The model under review builds one solid part; all positions refer to its coordinate system, in mm. A direction names the side the tool comes from. Coordinates: 2 decimals unless noted, no trailing zeros. Order: outer loops, then holes, each group sorted by start corner. A loop starts at its lowest first (then second) coordinate and runs counter-clockwise, first axis right, second up. Notation, with made-up numbers: M 18.5,29.25 L 42.5,29.25 A12 cw 42.5,41.25 Z; hole C 76,33 d9. An arc over 180 degrees is marked long. Write each question's results on one line, items separated by ' | '.
from build123d import *

# Parameters (mm, degrees)
SKETCH1_W           = 149.5
SKETCH1_H           = 70
BOSS_EXTRUDE1_DEPTH = 8
FILLET1_R           = 4
SKETCH6_W           = 147
SKETCH6_H           = 67.5
BOSS_EXTRUDE3_DEPTH = 5
FILLET2_R           = 4
SKETCH7_W           = 6.205469591
SKETCH7_H           = 30
BOSS_EXTRUDE4_DEPTH = 7
SKETCH8_R           = 1
CUT_EXTRUDE3_DEPTH  = 154.632882223
FILLET5_R           = 4
SKETCH9_W           = 90
SKETCH9_H           = 56
CUT_EXTRUDE4_DEPTH  = 7
SKETCH10_W          = 79
SKETCH10_H          = 56
CUT_EXTRUDE5_DEPTH  = 4
SKETCH11_W          = 66
SKETCH11_H          = 50
CUT_EXTRUDE6_DEPTH  = 85.478177656
SKETCH13_W          = 6
SKETCH13_H          = 50
BOSS_EXTRUDE5_DEPTH = 4
SKETCH14_R          = 1.692809378
CUT_EXTRUDE7_DEPTH  = 85.270768953
SKETCH15_W          = 6
SKETCH15_H          = 30
CUT_EXTRUDE8_DEPTH  = 2
CHAMFER2_SIZE       = 2
SKETCH16_R          = 3.75
CUT_EXTRUDE9_DEPTH  = 84.555744865
SKETCH17_W          = 12.5
SKETCH17_H          = 12.5
CUT_EXTRUDE10_DEPTH = 8
SKETCH20_W          = 24
SKETCH20_H          = 4
CUT_EXTRUDE12_DEPTH = 8
FILLET6_R           = 4
CHAMFER3_SIZE       = 2
SKETCH23_W          = 5.5
SKETCH23_H          = 43
CUT_EXTRUDE15_DEPTH = 4
FILLET7_R           = 1.5
CHAMFER6_SIZE       = 2
SKETCH26_W          = 27.5
SKETCH26_H          = 20
CUT_EXTRUDE16_DEPTH = 10
SKETCH27_W          = 27.410939183
SKETCH27_H          = 28.83766823
CUT_EXTRUDE17_DEPTH = 5
CHAMFER7_SIZE       = 3


with BuildPart() as part:
    # Sketch1 → Boss-Extrude1 (new body)
    with BuildSketch(Plane(origin=(0, 0, 0), x_dir=(1, 0, 0), z_dir=(0, 1, 0))):
        Rectangle(SKETCH1_W, SKETCH1_H)
    extrude(amount=BOSS_EXTRUDE1_DEPTH)

    # Fillet1
    fillet1_edges = [part.edges().sort_by_distance(p)[0] for p in [
        (74.75, 4, 35),
        (-74.75, 4, 35),
        (-74.75, 4, -35),
        (74.75, 4, -35),
    ]]
    fillet(fillet1_edges, radius=FILLET1_R)

    # Sketch6 → Boss-Extrude3 (add)
    with BuildSketch(Plane(origin=(0, 8, 0), x_dir=(1, 0, 0), z_dir=(0, 1, 0))):
        Rectangle(SKETCH6_W, SKETCH6_H)
    extrude(amount=BOSS_EXTRUDE3_DEPTH)

    # Fillet2
    fillet2_edges = [part.edges().sort_by_distance(p)[0] for p in [
        (73.5, 10.5, 33.75),
        (73.5, 10.5, -33.75),
        (-73.5, 10.5, -33.75),
        (-73.5, 10.5, 33.75),
    ]]
    fillet(fillet2_edges, radius=FILLET2_R)

    # Sketch7 → Boss-Extrude4 (add)
    with BuildSketch(Plane(origin=(0, 13, 0), x_dir=(1, 0, 0), z_dir=(0, 1, 0))):
        with Locations((-70.397265205, 0)):
            Rectangle(SKETCH7_W, SKETCH7_H)
        with Locations((70.397265205, 0)):
            Rectangle(SKETCH7_W, SKETCH7_H)
    extrude(amount=BOSS_EXTRUDE4_DEPTH)

    # Sketch8 → Cut-Extrude3 (cut, through all)
    with BuildSketch(Plane.ZY.offset(73.5)):
        with Locations((-7, 16)):
            Circle(SKETCH8_R)
        with Locations((7, 16)):
            Circle(SKETCH8_R)
    extrude(amount=-CUT_EXTRUDE3_DEPTH, mode=Mode.SUBTRACT)

    # Fillet5
    fillet5_edges = [part.edges().sort_by_distance(p)[0] for p in [
        (-70.397265204, 20, 15),
        (-70.397265204, 20, -15),
        (70.397265204, 20, -15),
        (70.397265204, 20, 15),
    ]]
    fillet(fillet5_edges, radius=FILLET5_R)

    # Sketch9 → Cut-Extrude4 (cut)
    with BuildSketch(Plane(origin=(0, 13, 0), x_dir=(1, 0, 0), z_dir=(0, 1, 0))):
        with Locations((-22, 0)):
            Rectangle(SKETCH9_W, SKETCH9_H)
    extrude(amount=-CUT_EXTRUDE4_DEPTH, mode=Mode.SUBTRACT)

    # Sketch10 → Cut-Extrude5 (cut)
    with BuildSketch(Plane(origin=(0, 6, 0), x_dir=(1, 0, 0), z_dir=(0, 1, 0))):
        with Locations((-22, 0)):
            Rectangle(SKETCH10_W, SKETCH10_H)
    extrude(amount=-CUT_EXTRUDE5_DEPTH, mode=Mode.SUBTRACT)

    # Sketch11 → Cut-Extrude6 (cut, through all)
    with BuildSketch(Plane(origin=(0, 2, 0), x_dir=(1, 0, 0), z_dir=(0, 1, 0))):
        with Locations((-18.5, 0)):
            Rectangle(SKETCH11_W, SKETCH11_H)
    extrude(amount=-CUT_EXTRUDE6_DEPTH, mode=Mode.SUBTRACT)

    # Sketch13 → Boss-Extrude5 (add)
    with BuildSketch(Plane(origin=(0, 13, 0), x_dir=(1, 0, 0), z_dir=(0, 1, 0))):
        with Locations((26, 0)):
            Rectangle(SKETCH13_W, SKETCH13_H)
    extrude(amount=BOSS_EXTRUDE5_DEPTH)

    # Sketch14 → Cut-Extrude7 (cut, through all)
    with BuildSketch(Plane(origin=(0, 17, 0), x_dir=(1, 0, 0), z_dir=(0, 1, 0))):
        with Locations(Location((26, 20, 0), (0, 0, 270))):
            Circle(SKETCH14_R)
        with Locations(Location((26, -20, 0), (0, 0, 90))):
            Circle(SKETCH14_R)
    extrude(amount=-CUT_EXTRUDE7_DEPTH, mode=Mode.SUBTRACT)

    # Sketch15 → Cut-Extrude8 (cut)
    with BuildSketch(Plane(origin=(0, 17, 0), x_dir=(1, 0, 0), z_dir=(0, 1, 0))):
        with Locations((26, 0)):
            Rectangle(SKETCH15_W, SKETCH15_H)
    extrude(amount=-CUT_EXTRUDE8_DEPTH, mode=Mode.SUBTRACT)

    # Chamfer2
    chamfer2_edges = [part.edges().sort_by_distance(p)[0] for p in [
        (26, 0, -21.692809378),
        (26, 0, 21.692809378),
    ]]
    chamfer(chamfer2_edges, length=CHAMFER2_SIZE)

    # Sketch16 → Cut-Extrude9 (cut, through all)
    with BuildSketch(Plane(origin=(0, 13, 0), x_dir=(1, 0, 0), z_dir=(0, 1, 0))):
        with Locations(Location((49.294530409, 0, 0), (0, 0, 270))):
            Circle(SKETCH16_R)
    extrude(amount=-CUT_EXTRUDE9_DEPTH, mode=Mode.SUBTRACT)

    # Sketch17 → Cut-Extrude10 (cut)
    with BuildSketch(Plane(origin=(0, 13, 0), x_dir=(1, 0, 0), z_dir=(0, 1, 0))):
        with Locations((49.294530409, 0)):
            Rectangle(SKETCH17_W, SKETCH17_H)
    extrude(amount=-CUT_EXTRUDE10_DEPTH, mode=Mode.SUBTRACT)

    # Sketch20 → Cut-Extrude12 (cut)
    with BuildSketch(Plane(origin=(0, 13, 0), x_dir=(1, 0, 0), z_dir=(0, 1, 0))):
        with Locations((-22, 30)):
            Rectangle(SKETCH20_W, SKETCH20_H)
        with Locations((-22, -30)):
            Rectangle(SKETCH20_W, SKETCH20_H)
    extrude(amount=-CUT_EXTRUDE12_DEPTH, mode=Mode.SUBTRACT)

    # Fillet6
    fillet6_edges = [part.edges().sort_by_distance(p)[0] for p in [
        (-34, 9, 32),
        (-10, 9, 32),
        (-10, 9, -32),
        (-34, 9, -32),
    ]]
    fillet(fillet6_edges, radius=FILLET6_R - 0.0001)  # a hair under: the kernel refuses the full size

    # Chamfer3
    chamfer3_edges = [part.edges().sort_by_distance(p)[0] for p in [
        (26, 17, 15),
        (26, 17, -15),
        (26, 17, -25),
        (26, 17, 25),
    ]]
    chamfer(chamfer3_edges, length=CHAMFER3_SIZE - 0.0001)  # a hair under: the kernel refuses the full size

    # Sketch23 → Cut-Extrude15 (cut)
    with BuildSketch(Plane(origin=(0, 6, 0), x_dir=(1, 0, 0), z_dir=(0, 1, 0))):
        with Locations((-64.25, 0)):
            Rectangle(SKETCH23_W, SKETCH23_H)
        with Locations((20.25, 0)):
            Rectangle(SKETCH23_W, SKETCH23_H)
    extrude(amount=-CUT_EXTRUDE15_DEPTH, mode=Mode.SUBTRACT)

    # Fillet7
    fillet7_edges = [part.edges().sort_by_distance(p)[0] for p in [
        (14.5, 1, -25),
        (14.5, 1, 25),
        (-51.5, 1, 25),
        (-51.5, 1, -25),
    ]]
    fillet(fillet7_edges, radius=FILLET7_R)

    # Chamfer6
    chamfer6_edges = [part.edges().sort_by_distance(p)[0] for p in [
        (-61.5, 4, 21.5),
        (-61.5, 4, -21.5),
        (17.5, 4, 21.5),
        (17.5, 4, -21.5),
    ]]
    chamfer(chamfer6_edges, length=CHAMFER6_SIZE)

    # Sketch26 → Cut-Extrude16 (cut)
    with BuildSketch(Plane(origin=(0, 13, 0), x_dir=(1, 0, 0), z_dir=(0, 1, 0))):
        with Locations((49.25, -21.75)):
            Rectangle(SKETCH26_W, SKETCH26_H)
        with Locations((49.25, 21.75)):
            Rectangle(SKETCH26_W, SKETCH26_H)
    extrude(amount=-CUT_EXTRUDE16_DEPTH, mode=Mode.SUBTRACT)

    # Sketch27 → Cut-Extrude17 (cut)
    with BuildSketch(Plane(origin=(0, 13, 0), x_dir=(1, 0, 0), z_dir=(0, 1, 0))):
        with Locations((49.294530409, 0)):
            Rectangle(SKETCH27_W, SKETCH27_H)
    extrude(amount=-CUT_EXTRUDE17_DEPTH, mode=Mode.SUBTRACT)

    # Chamfer7
    chamfer7_edges = [part.edges().sort_by_distance(p)[0] for p in [
        (-74.75, 0, 0),
        (74.75, 0, 0),
        (0, 0, 35),
        (0, 0, -35),
        (73.578427125, 0, 33.828427125),
        (73.578427125, 0, -33.828427125),
        (-73.578427125, 0, 33.828427125),
        (-73.578427125, 0, -33.828427125),
    ]]
    chamfer(chamfer7_edges, length=CHAMFER7_SIZE)


solid = part.part
1) Take a section at A-A on z = 20. Count the separate pieces of the cut face and the enclosed holes in it, plus the area to 3 significant figures.
Solutions:
separate pieces: 3 | enclosed holes: 0 | area: 487 mm2
2) For pin 1 (4 mm diameter, centred on x = -35.5, z = 25.5, fed in from +Y); pin 2 (1.5 mm diameter, centred on x = -22, y = 9.5, fed in from +Z); pin 3 (5 mm diameter, centred on y = 9.5, z = -10, fed in from -X); pin 4 (2 mm diameter, centred on x = 25, z = -16.5, fed in from +Y), all flat-tipped, find the tip position at first contact; note any pin that passes through.
Solutions:
pin 1: y = 2 | pin 2: z = 33.75 | pin 3: x = -74.75 | pin 4: y = 17
3) Take a section at B-B on x = -47. State the section outline as (y, z) points, plus the area to 4 significant figures.
Solutions:
outline: M 0,-32 L 3,-35 L 8,-35 L 8,-33.75 L 13,-33.75 L 13,-28 L 2,-28 L 2,-25 L 0,-25 Z; M 0,25 L 2,25 L 2,28 L 13,28 L 13,33.75 L 8,33.75 L 8,35 L 3,35 L 0,32 Z | area: 172.5 mm2
4) Take a section at D-D on x = -28. State the section outline as (y, z) points, plus the area to 4 significant figures.
Solutions:
outline: M 0,-32 L 3,-35 L 8,-35 L 8,-33.75 L 13,-33.75 L 13,-32 L 5,-32 L 5,-28 L 2,-28 L 2,-25 L 0,-25 Z; M 0,25 L 2,25 L 2,28 L 5,28 L 5,32 L 13,32 L 13,33.75 L 8,33.75 L 8,35 L 3,35 L 0,32 Z | area: 108.5 mm2
5) The part is to be moulded in two halves that separate along X. For faces 1 (the flat face through (-1, 5, 35)), 2 (the cylindrical face through (-73.609, 5.535, -33.797)), 3 (the flat face through (-67, 8, 0)), say which applies: pulls with the +X half, pulls with the -X half, needs draft (parallel to the pull), parting line crosses it, or undercut.
Solutions:
face 1: needs draft | face 2: pulls with the -X half | face 3: undercut
6) Take a section at C-C on x = 32.5. State the section outline as (y, z) points, plus the area to 4 significant figures.
Solutions:
outline: M 0,-32 L 3,-35 L 8,-35 L 8,-33.75 L 13,-33.75 L 13,33.75 L 8,33.75 L 8,35 L 3,35 L 0,32 Z | area: 888.5 mm2
7) For faces 4 (the flat face through (73.5, 13, 0)), 5 (the flat face through (26, 15, 0)), 6 (the conical face through (72.55, 1.52, 32.76)), list the 3-axis set-ups (+Z, -Z, +X, -X, +Y, -Y) from which the entire face can be reached by the end or side of a thin tool; tool diameter is ignored.
Solutions:
face 4: +Z, -Z, +X, +Y | face 5: +Y | face 6: +Z, +X, -Y
8) To check wall thickness, follow line 1 along X through (y, z) = (14.75, 14); line 2 along X through (y, z) = (12, -0.5); line 3 along X through (y, z) = (9, -20). State the ranges of each line that lie inside material, in increasing order.
Solutions:
line 1: -73.5 to -67.29, 23 to 29, 67.29 to 73.5 | line 2: -73.5 to -67, 23 to 35.59, 63 to 73.5 | line 3: -73.5 to -67, 23 to 24.31, 27.69 to 35.5, 63 to 73.5
